For this review, use the dimensioned drawing (mm, ordinates from the lowest corner) and the shaded views. A direction names the side the tool comes from. Coordinates: 2 decimals unless noted, no trailing zeros. Write each loop counter-clockwise with the first axis right and the second up, starting at its lowest first coordinate (ties: lowest second). Pieces come first, ordered by that corner, then holes. Notation, with made-up numbers: (72, 17.25) - (84, 17.25) arc R24 ccw to (84, 46.25) - close; hole circle Ø11 at (37.5, -9.5). An arc over 180 degrees is marked (long way). One line per item, written item: value.
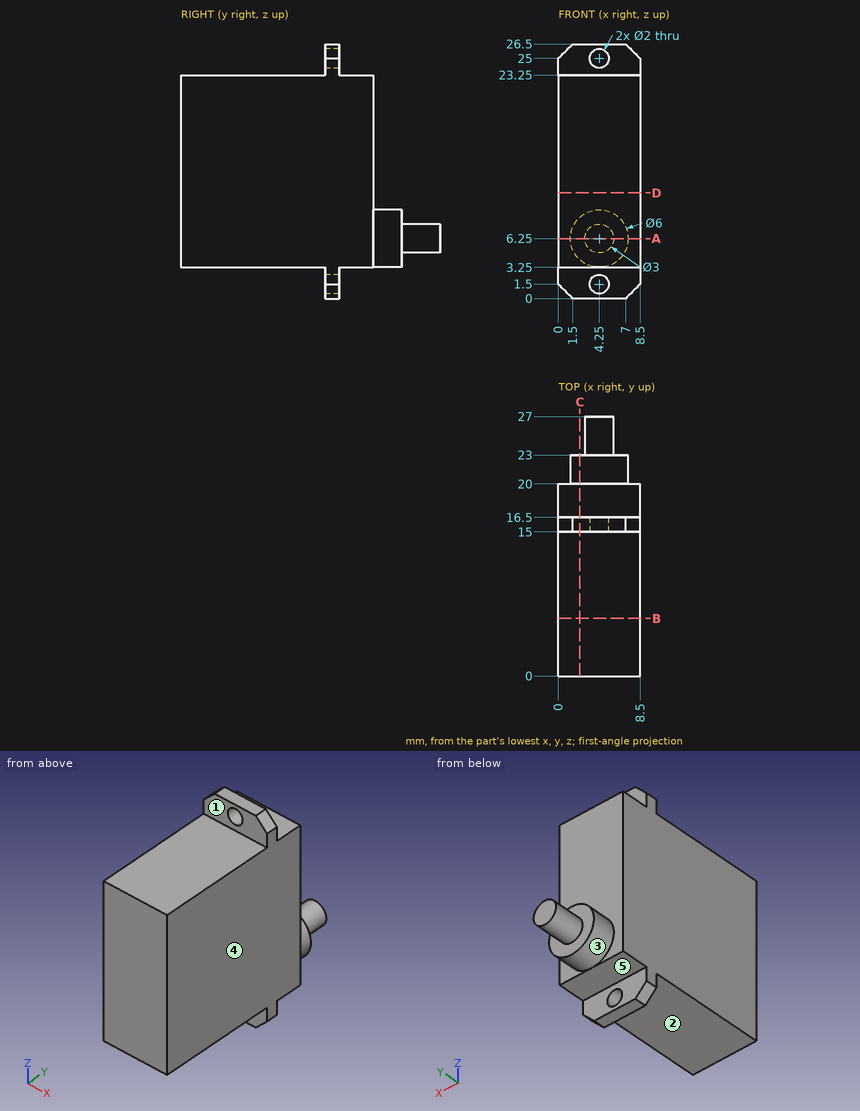
1. Consider section A-A, the plane z = 6.25. Write out the cut boundary in (x, y).
Answer block:
outline: (0, 0) - (8.5, 0) - (8.5, 20) - (7.25, 20) - (7.25, 23) - (5.75, 23) - (5.75, 27) - (2.75, 27) - (2.75, 23) - (1.25, 23) - (1.25, 20) - (0, 20) - close
2. Consider section C-C, the plane x = 2.25. Write out the cut boundary in (y, z), then the cut area to 3 significant figures.
Answer block:
outline: (0, 3.25) - (15, 3.25) - (15, 0) - (16.5, 0) - (16.5, 3.25) - (20, 3.25) - (20, 4.01) - (23, 4.01) - (23, 8.49) - (20, 8.49) - (20, 23.25) - (16.5, 23.25) - (16.5, 26.5) - (15, 26.5) - (15, 23.25) - (0, 23.25) - close
area: 423 mm^2
3. Consider section D-D, the plane z = 11. Write out the cut boundary in (x, y).
Answer block:
outline: (0, 0) - (8.5, 0) - (8.5, 20) - (0, 20) - close
4. For the marked faces 1, 2, 3, 4 and 5, list the 3-axis set-ups (+Z, -Z, +X, -X, +Y, -Y) from which the entire face can be reached by the end or side of a thin tool; tool diameter is ignored.
Answer block:
face 1: +Z, +X, -X, -Y
face 2: -Z, +X, -X, -Y
face 3: +Y
face 4: +Z, -Z, +X, +Y, -Y
face 5: -Z, +X, -X, +Y
5. Consider section B-B, the plane y = 6. Write out the cut boundary in (x, z).
Answer block:
outline: (0, 3.25) - (8.5, 3.25) - (8.5, 23.25) - (0, 23.25) - close
6. Insertion check: pin 1 Ø3 at (x, y) = (7, 18.5) entering from -Z; pin 2 Ø1 at (x, z) = (5.5, 2) entering from +Y; pin 3 Ø1.2 at (x, z) = (4.25, 25) entering from -Y; pin 4 Ø2 at (x, z) = (7, 6.5) entering from +Y. Each pin has a flat end and moves straight along its axis. Give the tip position at first contact, or say it passes through.
Answer block:
pin 1: stops at z = 3.25
pin 2: stops at y = 16.5
pin 3: passes through
pin 4: stops at y = 23
7. Wall thickness on line 1 along Z through (x, y) = (4.25, 15.6); line 2 along X through (y, z) = (15.3, 1.5); line 3 along Y through (x, z) = (5.75, 17.75): over which ranges is each line inside the solid? List them lowest first.
Answer block:
line 1: z = 0 to 0.5, 2.5 to 24, 26 to 26.5
line 2: x = 0 to 3.25, 5.25 to 8.5
line 3: y = 0 to 20
